Check sheet for the modelled part. Datum: model origin and axes. Units: mm. Round coordinates to 2 decimals unless told otherwise and drop trailing zeros. Order: outer loops, then holes, each group sorted by start corner. A loop starts at its lowest first (then second) coordinate and runs counter-clockwise, first axis right, second up.
```python
from build123d import *

# Parameters (mm, degrees)
EXTRUDE1_DEPTH          = 54.5
CUT_EXTRUDE1_DEPTH      = 55.854885702
CUT_EXTRUDE1_DEPTH_BACK = 55.854885702
SKETCH2_R               = 1.5


with BuildPart() as part:
    # Sketch1 → Extrude1 (new, symmetric)
    with BuildSketch(Plane(origin=(0, 0, 0), x_dir=(0, 0, -1), z_dir=(1, 0, 0))):
        with BuildLine():
            Line((-1.715977045, 5), (1.715977045, 5))
            ThreePointArc((1.715977045, 5), (2.824752941, 4.540729986), (3.284022955, 3.43195409))
            Line((3.284022955, 3.43195409), (3.284022955, -3.43195409))
            ThreePointArc((3.284022955, -3.43195409), (2.824752941, -4.540729986), (1.715977045, -5))
            Line((1.715977045, -5), (-1.715977045, -5))
            ThreePointArc((-1.715977045, -5), (-2.672673527, -4.674330771), (-3.23197526, -3.832600305))
            ThreePointArc((-3.23197526, -3.832600305), (-3.383560587, -3.204564402), (-3.507961213, -2.570583572))
            ThreePointArc((-3.507961213, -2.570583572), (-3.356955711, -1.900195953), (-3.674237451, -1.290643232))
            ThreePointArc((-3.674237451, -1.290643232), (-3.698584955, -0.968220458), (-3.715977045, -0.645347786))
            ThreePointArc((-3.715977045, -0.645347786), (-3.479865934, 0), (-3.715977045, 0.645347786))
            ThreePointArc((-3.715977045, 0.645347786), (-3.698584955, 0.968220458), (-3.674237451, 1.290643232))
            ThreePointArc((-3.674237451, 1.290643232), (-3.356955711, 1.900195953), (-3.507961213, 2.570583572))
            ThreePointArc((-3.507961213, 2.570583572), (-3.383560587, 3.204564402), (-3.23197526, 3.832600305))
            ThreePointArc((-3.23197526, 3.832600305), (-2.672673527, 4.674330771), (-1.715977045, 5))
        make_face()
        with BuildLine():
            Line((-1.715977045, 4), (1.715977045, 4))
            ThreePointArc((1.715977045, 4), (2.11764616, 3.833623205), (2.284022955, 3.43195409))
            Line((2.284022955, 3.43195409), (2.284022955, -3.43195409))
            ThreePointArc((2.284022955, -3.43195409), (2.11764616, -3.833623205), (1.715977045, -4))
            Line((1.715977045, -4), (-1.715977045, -4))
            ThreePointArc((-1.715977045, -4), (-2.062553328, -3.882021902), (-2.265167971, -3.577093618))
            ThreePointArc((-2.265167971, -3.577093618), (-2.729865934, 0), (-2.265167971, 3.577093618))
            ThreePointArc((-2.265167971, 3.577093618), (-2.062553328, 3.882021902), (-1.715977045, 4))
        make_face(mode=Mode.SUBTRACT)
    extrude(amount=EXTRUDE1_DEPTH, both=True)

    # Sketch2 → Cut-Extrude1 (cut, two sides: drawn at the far end of the back side and taken through both)
    with BuildSketch(Plane(origin=(0, 0, 0), x_dir=(1, 0, 0), z_dir=(0, 1, 0)).offset(-CUT_EXTRUDE1_DEPTH_BACK)):
        with Locations(Location((-51.285, 0, 0), (0, 0, 270))):
            Circle(SKETCH2_R)
        with Locations(Location((51.285, 0, 0), (0, 0, 90))):
            Circle(SKETCH2_R)
    extrude(amount=CUT_EXTRUDE1_DEPTH + CUT_EXTRUDE1_DEPTH_BACK, mode=Mode.SUBTRACT)


solid = part.part
```
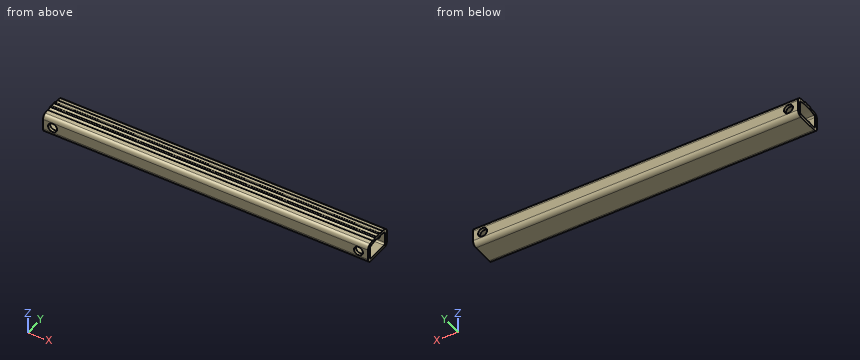
Item 1: Go/stop test with flat-tipped pins: P1, Ø2.5, axis at x = -51.285, z = 0, coming from the +Y side; P2, Ø2, axis at x = -2.5, y = 2, coming from the +Z side. Record where each tip stops, or that it passes through.
Answer:
P1: passes through
P2: stops at z = 3.7
Item 2: Sectioned sample at A-A (z = 0). Record the cut outline in (x, y) (3 decimals).
Answer:
outline: (-54.5, -5) - (-52.785, -5) - (-52.785, -4) - (-54.5, -4) - close; (-54.5, 4) - (-52.785, 4) - (-52.785, 5) - (-54.5, 5) - close; (-49.785, -5) - (49.785, -5) - (49.785, -4) - (-49.785, -4) - close; (-49.785, 4) - (49.785, 4) - (49.785, 5) - (-49.785, 5) - close; (52.785, -5) - (54.5, -5) - (54.5, -4) - (52.785, -4) - close; (52.785, 4) - (54.5, 4) - (54.5, 5) - (52.785, 5) - close
Item 3: Sectioned sample at B-B (x = -18.5). Record the cut outline in (y, z).
Answer:
outline: (-5, -1.72) arc R1.57 ccw to (-3.43, -3.28) - (3.43, -3.28) arc R1.57 ccw to (5, -1.72) - (5, 1.72) arc R1.57 ccw to (3.83, 3.23) arc R15 ccw to (2.57, 3.51) arc R1 cw to (1.29, 3.67) arc R15 ccw to (0.65, 3.72) arc R1 cw to (-0.65, 3.72) arc R15 ccw to (-1.29, 3.67) arc R1 cw to (-2.57, 3.51) arc R15 ccw to (-3.83, 3.23) arc R1.57 ccw to (-5, 1.72) - close; hole (-4, -1.72) arc R0.57 ccw to (-3.43, -2.28) - (3.43, -2.28) arc R0.57 ccw to (4, -1.72) - (4, 1.72) arc R0.57 ccw to (3.58, 2.27) arc R14 ccw to (-3.58, 2.27) arc R0.57 ccw to (-4, 1.72) - close
Item 4: Scan lines: line 1 along X through (y, z) = (4.5, 0) (3 decimals); line 2 along Y through (x, z) = (47, 0.5); line 3 along X through (y, z) = (-4.25, -1.25). Record each from-to range of solid material in increasing order.
Answer:
line 1: x = -54.5 to -52.785, -49.785 to 49.785, 52.785 to 54.5
line 2: y = -5 to -4, 4 to 5
line 3: x = -54.5 to -52.11, -50.46 to 50.46, 52.11 to 54.5
